from build123d import *

# Parameters (mm, degrees)
AUFSATZ_LINEAR_AUSTRAGEN1_DEPTH = 2


with BuildPart() as part:
    # Skizze1 → Aufsatz-Linear austragen1 (new body)
    with BuildSketch(Plane(origin=(0, 0, 0), x_dir=(0, 1, 0), z_dir=(0, 0, 1))):
        Polygon((-5.5, 4), (5.5, 4), (3.843145751, 0), (-3.843145751, 0), align=None)
    aufsatz_linear_austragen1 = extrude(amount=AUFSATZ_LINEAR_AUSTRAGEN1_DEPTH)

    # Spiegeln1: Aufsatz-Linear austragen1 across plane
    add(aufsatz_linear_austragen1.mirror(Plane(origin=(0, 3.843145751, 2), x_dir=(0, 0, 1), z_dir=(-1, 0, 0))))


solid = part.part
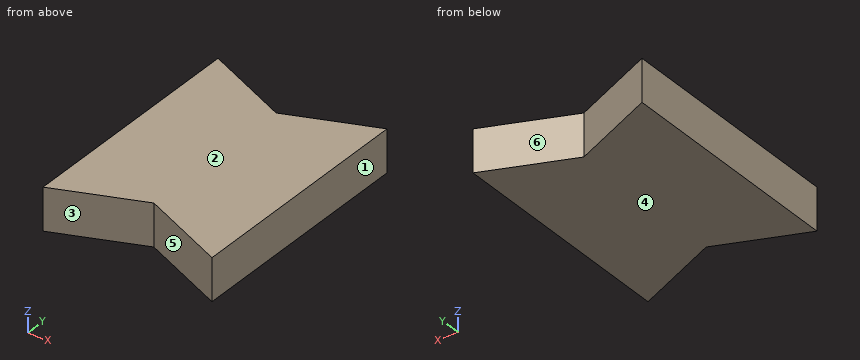
Model file for the job. Use its own axes, mm. Face numbers are marked on the shaded views. A direction names the side the tool comes from. Coordinates: 2 decimals unless noted, no trailing zeros. Order: outer loops, then holes, each group sorted by start corner. A loop starts at its lowest first (then second) coordinate and runs counter-clockwise, first axis right, second up. Notation, with made-up numbers: (9.5, 72) -> (64.5, 72) arc R8 ccw to (64.5, 79) -> close; hole circle Ø10 at (0, -35). An arc over 180 degrees is marked (long way). Return JSON: item names as keys, results as strings. Group by question number.
Item 1: Saw through at B-B on x = -3.5. Write the cut outline in (y, z), then the cut area to 3 significant figures.
Item 2: Saw through at A-A on z = 0.2. Write the cut outline in (x, y), then the cut area to 3 significant figures.
Item 3: Wall check: line 1 along X through (y, z) = (-5, 1.1); line 2 along Y through (x, z) = (2, 0.5); line 3 along Y through (x, z) = (2.25, 1.55). Give the ranges that are in metal, low to high. Write a range as [from, to].
Item 4: Pull direction X, two halves, no side cores. Call the marked faces 1, 2 and 3: pulls with the +X half, pulls with the -X half, needs draft (parallel to the pull), parting line crosses it, or undercut.
Item 5: Saw through at C-C on x = -2. Write the cut outline in (y, z).
Item 6: Tool access for the marked faces 4, 5 and 6: list every direction of +Z, -Z, +X, -X, +Y, -Y with a clear straight run to the whole face (end or side of a thin tool).
Values found:
{
 "1": {"outline": "(-5.29, 0) -> (5.29, 0) -> (5.29, 2) -> (-5.29, 2) -> close", "area": "21.2 mm2"},
 "2": {"outline": "(-4, -5.5) -> (0, -3.84) -> (4, -5.5) -> (4, 5.5) -> (0, 3.84) -> (-4, 5.5) -> close", "area": "74.7 mm2"},
 "3": {"line 1": "x = [-4, -2.79], [2.79, 4]", "line 2": "y = [-4.67, 4.67]", "line 3": "y = [-4.78, 4.78]"},
 "4": {"face 1": "pulls with the +X half", "face 2": "needs draft", "face 3": "undercut"},
 "5": {"outline": "(-4.67, 0) -> (4.67, 0) -> (4.67, 2) -> (-4.67, 2) -> close"},
 "6": {"face 4": "-Z, +X, -X, +Y, -Y", "face 5": "+Z, -Z, -Y", "face 6": "+Z, -Z, +Y"}
}
